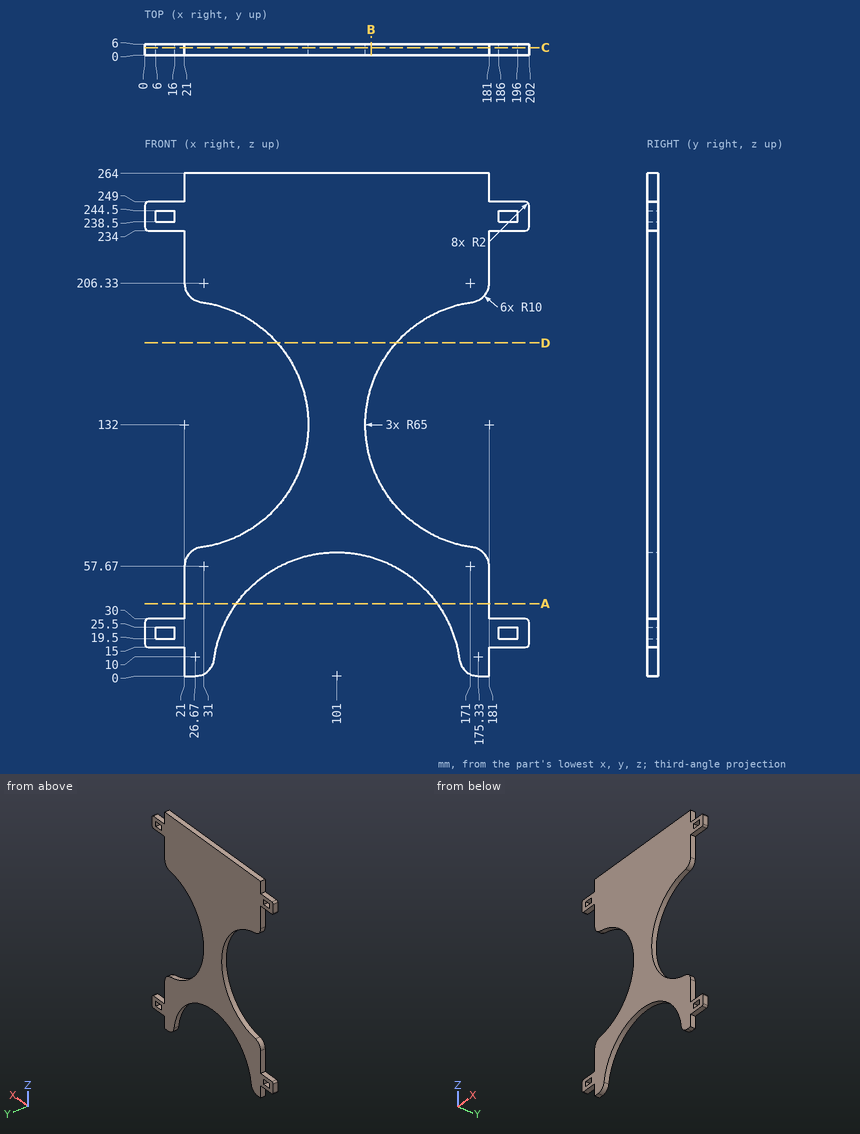
Could you check a few things on this drawing? It's one solid part, dimensions in mm from its lowest x, y, z. Coordinates: 2 decimals unless noted, no trailing zeros. Write each loop counter-clockwise with the first axis right and the second up, starting at its lowest first coordinate (ties: lowest second). Pieces come first, ordered by that corner, then holes.
1) If we section it at A-A (z = 38): List the corners of the cut face in (x, y) for me (1 decimal).
Filled in:
outline: (21, 0) - (48.3, 0) - (48.3, 6) - (21, 6) - close; (153.7, 0) - (181, 0) - (181, 6) - (153.7, 6) - close
2) If we section it at D-D (z = 175): List the corners of the cut face in (x, y) for me, plus the area to 3 significant figures.
Filled in:
outline: (69.74, 0) - (132.26, 0) - (132.26, 6) - (69.74, 6) - close
area: 375 mm2
3) If we section it at B-B (x = 119): List the corners of the cut face in (y, z) for me, plus the area to 3 significant figures.
Filled in:
outline: (0, 62.46) - (6, 62.46) - (6, 112.48) - (0, 112.48) - close; (0, 151.52) - (6, 151.52) - (6, 264) - (0, 264) - close
area: 975 mm2
4) I'm going to push flat-ended pins straight in: pin 1 (3 mm diameter, centred on x = 192, y = 4.5, fed in from +Z); pin 2 (1.5 mm diameter, centred on x = 154, y = 4, fed in from -Z); pin 3 (1.8 mm diameter, centred on x = 11.5, y = 4, fed in from -Z). Where does each tip first touch, or does it pass through?
Filled in:
pin 1: stops at z = 249
pin 2: stops at z = 36.55
pin 3: stops at z = 15
5) If I drill on line 1 (X direction, y = 1.85, z = 239.5); line 2 (X direction, y = 4.3, z = 132.5); line 3 (Z direction, x = 51, y = 1.5) (1 decimal), over which ranges is the centre line in solid material (lowest first)?
Filled in:
line 1: x = 0 to 6, 16 to 186, 196 to 202
line 2: x = 86 to 116
line 3: z = 41.5 to 74.3, 189.7 to 264
6) If we section it at C-C (y = 4.1): Count the separate pieces of the cut face and the enclosed holes in it, plus the area to 3 significant figures.
Filled in:
separate pieces: 1
enclosed holes: 4
area: 23,200 mm2
